Geometry check sheet. Reference: drawing and pictorial views, mm from the part's lowest x, y, z. Round coordinates to 2 decimals unless told otherwise and drop trailing zeros. Order: outer loops, then holes, each group sorted by start corner. A loop starts at its lowest first (then second) coordinate and runs counter-clockwise, first axis right, second up.
(1) Sectioned sample at B-B, the plane y = 108. Enter the section's corners in (x, z).
(2) Depth check by flat-ended pin: pin 1 (6 mm diameter, centred on y = 46, z = 19, fed in from -X); pin 2 (6 mm diameter, centred on y = 72, z = 17.5, fed in from +X); pin 3 (12 mm diameter, centred on x = 61.5, z = 28.5, fed in from +Y); pin 4 (12 mm diameter, centred on x = 125, y = 24.5, fed in from -Z). Enter the tip coordinate at first touch or a pass-through.
(3) Sectioned sample at A-A, the plane x = 81. Enter the section's corners in (y, z).
(4) Mould release check, pull along Y, two halves, no side actions. Record for the marked faces 1 and 2: released by +Y, released by -Y, zero draft, split by the parting line, or undercut.
(5) Thickness scan on probe 1 along X at (y, z) = (148, 36.5) (1 decimal); probe 2 along X at (y, z) = (18.5, 29) (1 decimal); probe 3 along Y at (x, z) = (23, 12.5). Record the ranges inside material, lowest first.
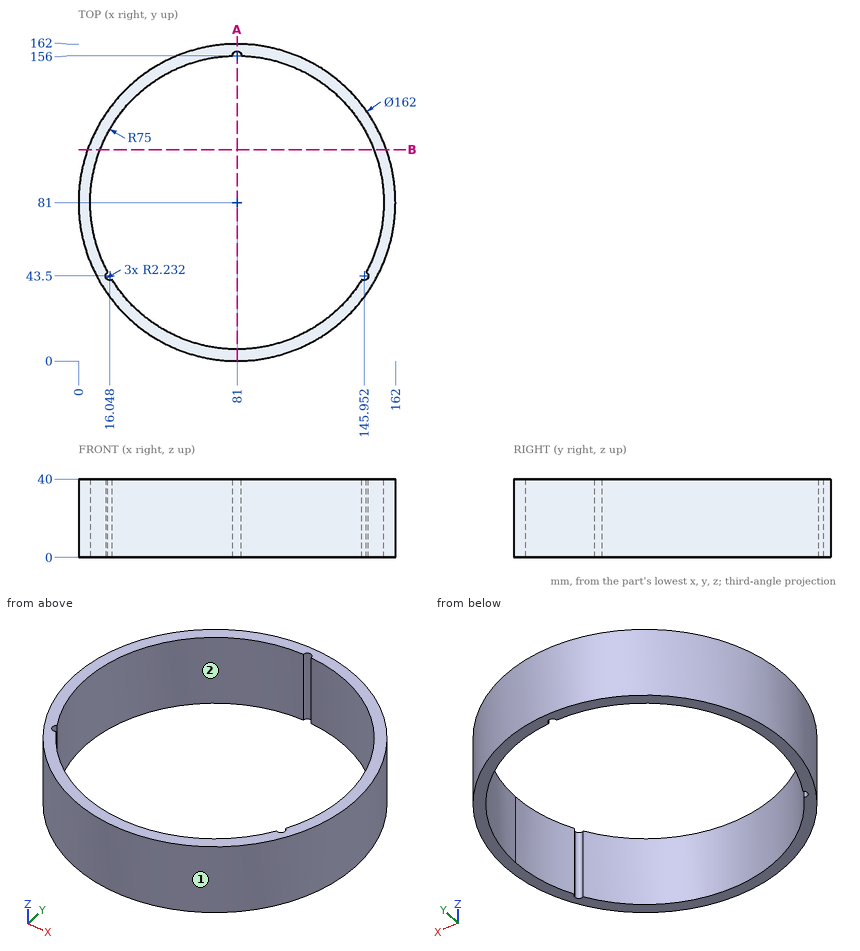
Derived:
1. outline: (4.63, 0) - (11.03, 0) - (11.03, 40) - (4.63, 40) - close; (150.97, 0) - (157.37, 0) - (157.37, 40) - (150.97, 40) - close
2. pin 1: stops at x = 6.59
2. pin 2: stops at x = 161.78
2. pin 3: stops at y = 160.87
2. pin 4: stops at z = 0
3. outline: (0, 0) - (6, 0) - (6, 40) - (0, 40) - close; (158.23, 0) - (162, 0) - (162, 40) - (158.23, 40) - close
4. face 1: split by the parting line
4. face 2: undercut
5. probe 1: x = 35.5 to 47.3, 114.7 to 126.5
5. probe 2: x = 29.5 to 39.5, 122.5 to 132.5
5. probe 3: y = 24.46 to 33.45, 128.55 to 137.54
